```python
from build123d import *

# Parameters (mm, degrees)
SKETCH2_R               = 19.5
BOSS_EXTRUDE1_DEPTH     = 12
SKETCH3_R               = 11
CUT_EXTRUDE2_DEPTH      = 47
CUT_EXTRUDE2_DEPTH_BACK = 47
SKETCH7_W               = 36
SKETCH7_H               = 8
CUT_EXTRUDE4_DEPTH      = 47.0000001


with BuildPart() as part:
    # Sketch1 → Revolve1 (revolve)
    with BuildSketch(Plane(origin=(0, 0, 0), x_dir=(1, 0, 0), z_dir=(0, 1, 0))):
        Polygon((0, 41.324206049), (46, 41.324206049), (46, 39.324206049), (42, 39.324206049), (42, 36.324206049), (46, 36.324206049), (46, 34.324206049), (42, 34.324206049), (42, 31.324206049), (46, 31.324206049), (46, 29.324206049), (42, 29.324206049), (42, 26.324206049), (46, 26.324206049), (46, 24.324206049), (42, 24.324206049), (42, 21.324206049), (46, 21.324206049), (46, -17.675793951), (42, -17.675793951), (42, -19.675793951), (46, -19.675793951), (46, -24.675793951), (37, -24.675793951), (37, 22.858692986), (37, 37.324206049), (0, 37.324206049), align=None)
    revolve(axis=Axis((0, 0, 0), (0, 0, -1)))

    # Sketch2 → Boss-Extrude1 (add)
    with BuildSketch(Plane(origin=(0, 25, 0), x_dir=(1, 0, 0), z_dir=(0, 1, 0))):
        with Locations((0, 2.324206049)):
            Circle(SKETCH2_R)
    boss_extrude1 = extrude(amount=BOSS_EXTRUDE1_DEPTH)

    # Mirror1: Boss-Extrude1 across plane
    add(boss_extrude1.mirror(Plane.ZX))

    # Sketch3 → Cut-Extrude2 (cut, two sides)
    with BuildSketch(Plane(origin=(0, 0, 0), x_dir=(1, 0, 0), z_dir=(0, 1, 0))) as cut_extrude2_sk:
        with Locations((0, 2.324206049)):
            Circle(SKETCH3_R)
    extrude(amount=CUT_EXTRUDE2_DEPTH, mode=Mode.SUBTRACT)
    extrude(cut_extrude2_sk.sketch, amount=-CUT_EXTRUDE2_DEPTH_BACK, mode=Mode.SUBTRACT)

    # Sketch7 → Cut-Extrude4 (cut, symmetric)
    with BuildSketch(Plane(origin=(0, 0, 0), x_dir=(0, 0, -1), z_dir=(1, 0, 0))):
        with Locations((2.324206049, 46)):
            Rectangle(SKETCH7_W, SKETCH7_H)
    cut_extrude4 = extrude(amount=CUT_EXTRUDE4_DEPTH, both=True, mode=Mode.SUBTRACT)

    # Mirror2: Cut-Extrude4 across plane
    add(cut_extrude4.mirror(Plane.ZX), mode=Mode.SUBTRACT)


solid = part.part
```
For this review, take the finished solid that the model builds, in its own axes (mm). A direction names the side the tool comes from. Round coordinates to 2 decimals unless told otherwise and drop trailing zeros. Order: outer loops, then holes, each group sorted by start corner. A loop starts at its lowest first (then second) coordinate and runs counter-clockwise, first axis right, second up.
Q1. Machinability: for faces 4 (the flat face through (8, 25, 6)), 5 (the flat face through (-1, -1, -37.324)), 6 (the flat face through (0, 44, 15.676)), 7 (the flat face through (0, -44, -20.324)), which of the approach directions +Z, -Z, +X, -X, +Y, -Y give a long, thin tool a straight path to every point of the face, cutting with its end or side? Answer none if there is none.
Findings below:
face 4: +Z
face 5: none
face 6: +X, -X, +Y
face 7: +X, -X, -Y
Q2. We need section B-B, the plane x = 0. State how many separate pieces and enclosed holes the cut face has, plus the area to 3 significant figures.
Findings below:
separate pieces: 3
enclosed holes: 0
area: 1,270 mm2
Q3. We need section C-C, the plane z = -19. Give the boundary of the cut face in (x, y), plus the area to 3 significant figures.
Findings below:
outline: (-18.76, -42) - (18.76, -42) arc R46 ccw to (18.76, 42) - (-18.76, 42) arc R46 ccw to start; hole (-10.11, -35.59) - (-10.11, -25) - (10.11, -25) - (10.11, -35.59) arc R37 ccw to (10.11, 35.59) - (10.11, 25) - (-10.11, 25) - (-10.11, 35.59) arc R37 ccw to start
area: 2,610 mm2
Q4. Mouldability with a two-part tool opening along Z and no side actions: class faces 1 (the flat face through (1, -1, -41.324)), 2 (the cylindrical face through (-5.99, -45.61, 22.21)), 3 (the cylindrical face through (40.06, -12.62, -27.8)) as pulls with the +Z half, pulls with the -Z half, needs draft (parallel to the pull), parting line crosses it, or undercut.
Findings below:
face 1: pulls with the -Z half
face 2: needs draft
face 3: undercut
Q5. Insertion check: P1, Ø19.5, axis at x = -4, z = 7.5, coming from the -Y side; P2, Ø4, axis at y = 10.5, z = -7, coming from the -X side; P3, Ø11, axis at x = 9, z = -6, coming from the +Y side. Each pin has a flat end and moves straight along its axis. Give the tip position at first contact, or say it passes through.
Findings below:
P1: stops at y = -46
P2: stops at x = -45.21
P3: stops at y = 42
Q6. Wall thickness on line 1 (Z direction, x = 0, y = -34.5); line 2 (X direction, y = 0, z = 7); line 3 (Y direction, x = 1.5, z = 11.5): over which ranges is each line inside the solid? List them lowest first.
Findings below:
line 1: z = -41.32 to -37.32, -21.82 to -13.32, 8.68 to 17.18
line 2: x = -46 to -37, 37 to 46
line 3: y = -42 to -25, 25 to 42
Q7. We need section A-A, the plane z = 4. Give the boundary of the cut face in (x, y), plus the area to 3 significant figures.
Findings below:
outline: (-18.76, -42) - (-9, -42) - (-9, -25) - (-18.45, -25) - (-18.45, -32.07) arc R37 cw to (-18.45, 32.07) - (-18.45, 25) - (-9, 25) - (-9, 42) - (-18.76, 42) arc R46 ccw to start; (9, -42) - (18.76, -42) arc R46 ccw to (18.76, 42) - (9, 42) - (9, 25) - (18.45, 25) - (18.45, 32.07) arc R37 cw to (18.45, -32.07) - (18.45, -25) - (9, -25) - close
area: 2,300 mm2
